Can you work these out from the model? Positions are in its coordinate system, mm. Give positions to 0.01 mm unless a question says otherwise; leave off trailing zeros. Write each loop counter-clockwise with the first axis right and the second up, starting at its lowest first coordinate (ties: lowest second). Pieces come first, ordered by that corner, then holes. Notation, with made-up numbers: (56.25, -15) -> (98.25, -15) arc R30 cw to (98.25, 23) -> close; hole circle Ø7 at (38.25, 32). An arc over 180 degrees is marked (long way). Answer as CSV lines item,"result". Start each with the question number.
1. If we section it at C-C on z = 1.3: Write out the boundary of the cut face in (x, y).
2. If we section it at B-B on y = -19.5: Write out the boundary of the cut face in (x, z).
3. If we section it at A-A on x = 0: Write out the boundary of the cut face in (y, z), plus the area to 3 significant figures.
4. If we section it at D-D on x = 20: Write out the boundary of the cut face in (y, z), plus the area to 3 significant figures.
5. If we mould it in two halves opening along X, with no side actions, what happens to faces 1 (the face through (-11, 20, 0)), 2 (the face through (10.382, -19.961, 0.789))? For each: pulls with the +X half, pulls with the -X half, needs draft (parallel to the pull), parting line crosses it, or undercut.
6. I'm going to push a flat-ended pin straight in: P1, Ø2.5, axis at x = 0, y = -40.91, coming from the -Z side. Where does the tip first touch, or does it pass through?
7. I need wall thicknesses on line 1 (Y direction, x = 0, z = 1.25); line 2 (X direction, y = 33.5, z = 1); line 3 (Y direction, x = -1.5, z = 0.7). Which ranges of each line are inside material? Lowest first, please. Write a range as [from, to].
```python
from build123d import *

# Parameters (mm, degrees)
F0_R     = 22.5
F1_DEPTH = 1.6


with BuildPart() as f1:
    # F0 (on Top) → F1 (new body)
    with BuildSketch(Plane.XY):
        with BuildLine():
            ThreePointArc((23.5, -37.7888872554), (38.8973006776, -21.6159663212), (44.5, 0))
            ThreePointArc((44.5, 0), (-21.6159663212, 38.8973006776), (-23.5, -37.7888872554))
            Line((-23.5, -37.7888872554), (-23.5, 31.8375))
            ThreePointArc((-23.5, 31.8375), (-24.666726189, 34.654226189), (-21.85, 33.4875))
            Line((-21.85, 33.4875), (21.85, 33.4875))
            ThreePointArc((21.85, 33.4875), (23.5, 35.1375), (25.15, 33.4875))
            ThreePointArc((25.15, 33.4875), (24.666726189, 32.320773811), (23.5, 31.8375))
            Line((23.5, 31.8375), (23.5, -37.7888872554))
        make_face()
        with BuildLine():
            Line((-23.5, 31.8375), (-23.5, -37.7888872554))
            ThreePointArc((-23.5, -37.7888872554), (-20.5617909506, -39.4647026202), (-17.504780597, -40.9125))
            Line((-17.504780597, -40.9125), (-1.65, -40.9125))
            ThreePointArc((-1.65, -40.9125), (0, -39.2625), (1.65, -40.9125))
            Line((1.65, -40.9125), (17.504780597, -40.9125))
            ThreePointArc((17.504780597, -40.9125), (20.5617909506, -39.4647026202), (23.5, -37.7888872554))
            Line((23.5, -37.7888872554), (23.5, 31.8375))
            ThreePointArc((23.5, 31.8375), (22.333273811, 32.320773811), (21.85, 33.4875))
            Line((21.85, 33.4875), (-21.85, 33.4875))
            ThreePointArc((-21.85, 33.4875), (-22.333273811, 32.320773811), (-23.5, 31.8375))
        make_face()
        Circle(F0_R, mode=Mode.SUBTRACT)
        with BuildLine():
            Line((-1.65, -40.9125), (-17.504780597, -40.9125))
            ThreePointArc((-17.504780597, -40.9125), (0, -44.5), (17.504780597, -40.9125))
            Line((17.504780597, -40.9125), (1.65, -40.9125))
            ThreePointArc((1.65, -40.9125), (0, -42.5625), (-1.65, -40.9125))
        make_face()
    extrude(amount=F1_DEPTH)


solid = f1.part
```
Computed values:
1,outline,"circle Ø89 at (0, 0); hole circle Ø3.3 at (-23.5, 33.49); hole circle Ø45 at (0, 0); hole circle Ø3.3 at (0, -40.91); hole circle Ø3.3 at (23.5, 33.49)"
2,outline,"(-40, 0) -> (-11.22, 0) -> (-11.22, 1.6) -> (-40, 1.6) -> close; (11.22, 0) -> (40, 0) -> (40, 1.6) -> (11.22, 1.6) -> close"
3,outline,"(-44.5, 0) -> (-42.56, 0) -> (-42.56, 1.6) -> (-44.5, 1.6) -> close; (-39.26, 0) -> (-22.5, 0) -> (-22.5, 1.6) -> (-39.26, 1.6) -> close; (22.5, 0) -> (44.5, 0) -> (44.5, 1.6) -> (22.5, 1.6) -> close"
3,area,"65.1 mm2"
4,outline,"(-39.75, 0) -> (-10.31, 0) -> (-10.31, 1.6) -> (-39.75, 1.6) -> close; (10.31, 0) -> (39.75, 0) -> (39.75, 1.6) -> (10.31, 1.6) -> close"
4,area,"94.2 mm2"
5,face 1,"needs draft"
5,face 2,"undercut"
6,P1,"passes through"
7,line 1,"y = [-44.5, -42.56], [-39.26, -22.5], [22.5, 44.5]"
7,line 2,"x = [-29.29, -25.15], [-21.85, 21.85], [25.15, 29.29]"
7,line 3,"y = [-44.47, -41.6], [-40.23, -22.45], [22.45, 44.47]"
